Work out the finished part from the listing and answer in its coordinate system (mm). Face numbers are marked on the shaded views. A direction names the side the tool comes from. Coordinates: 2 decimals unless noted, no trailing zeros. Write each loop counter-clockwise with the first axis right and the second up, starting at its lowest first coordinate (ties: lowest second). Pieces come first, ordered by that corner, then holes. Notation, with made-up numbers: (83, -34) - (119, -34) arc R27 cw to (119, 1) - close; hole circle Ø8 at (-39, -2.5). An arc over 180 degrees is marked (long way). Use CSV: the item, a comma, the result in double quotes. Start each with the question number.
from build123d import *

# Parameters (mm, degrees)
SKETCH2_R           = 16
BOSS_EXTRUDE1_DEPTH = 5
SKETCH3_R           = 7.5
BOSS_EXTRUDE2_DEPTH = 19
SKETCH4_R           = 4
CUT_EXTRUDE1_DEPTH  = 50
SKETCH5_R           = 2
CUT_EXTRUDE2_DEPTH  = 50


with BuildPart() as part:
    # Sketch2 → Boss-Extrude1 (new body)
    with BuildSketch(Plane(origin=(0, 0, 0), x_dir=(1, 0, 0), z_dir=(0, 1, 0))):
        Circle(SKETCH2_R)
    extrude(amount=BOSS_EXTRUDE1_DEPTH)

    # Sketch3 → Boss-Extrude2 (add)
    with BuildSketch(Plane(origin=(0, 5, 0), x_dir=(1, 0, 0), z_dir=(0, 1, 0))):
        Circle(SKETCH3_R)
    extrude(amount=BOSS_EXTRUDE2_DEPTH)

    # Sketch4 → Cut-Extrude1 (cut)
    with BuildSketch(Plane(origin=(0, 24, 0), x_dir=(1, 0, 0), z_dir=(0, 1, 0))):
        Circle(SKETCH4_R)
    extrude(amount=-CUT_EXTRUDE1_DEPTH, mode=Mode.SUBTRACT)

    # Sketch5 → Cut-Extrude2 (cut)
    with BuildSketch(Plane(origin=(0, 5, 0), x_dir=(1, 0, 0), z_dir=(0, 1, 0))):
        with Locations((0, 12)):
            Circle(SKETCH5_R)
        with Locations((0, -12)):
            Circle(SKETCH5_R)
        with Locations((-12, 0)):
            Circle(SKETCH5_R)
        with Locations((12, 0)):
            Circle(SKETCH5_R)
    extrude(amount=-CUT_EXTRUDE2_DEPTH, mode=Mode.SUBTRACT)


solid = part.part
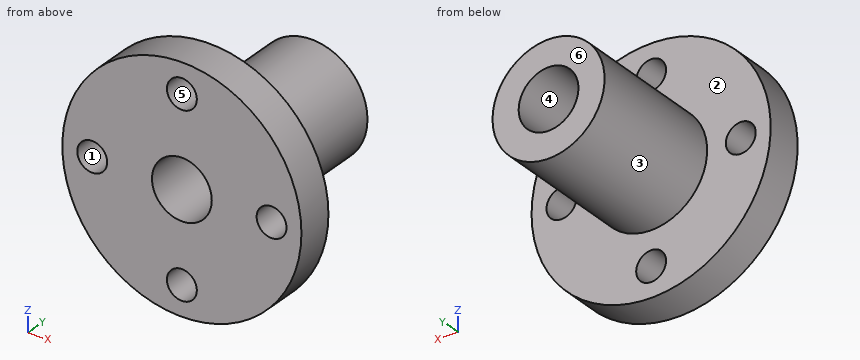
Item 1: Each of these flat-tipped pins is pushed along its axis until it touches: pin 1 (6 mm diameter, centred on x = 7.5, y = 19, fed in from -Z); pin 2 (8 mm diameter, centred on x = -7, y = 14, fed in from -Z); pin 3 (4.5 mm diameter, centred on x = 0, z = -12, fed in from +Y). Where does it stop, or does it pass through?
Item 2: Straight lines are drawn through the part: probe 1 along X at (y, z) = (2.85, 0); probe 2 along X at (y, z) = (6, 0). For each, find the intervals that lie inside material, in ascending order. Write a range as [from, to].
Item 3: A cutting plane is placed at C-C (x = -12). Determine the outline of the cut face in (y, z).
Item 4: Which of the six approach directions +Z, -Z, +X, -X, +Y, -Y give full straight-line access (tool end or side, diameter ignored) to the marked faces 1 and 2?
Item 5: A cutting plane is placed at A-A (x = 0). Determine the outline of the cut face in (y, z).
Item 6: A cutting plane is placed at D-D (y = 7.75). Determine the outline of the cut face in (x, z), then the cut area to 3 significant figures.
Item 7: A cutting plane is placed at B-B (z = 0.5). Determine the outline of the cut face in (x, y), then the cut area to 3 significant figures.
Item 8: Determine the mould class of the marked faces 3, 4, 5 and 6 for opening direction X: +X half, -X half, draft (parallel to the pull), parting line (faces both ways), or undercut.
Calculated:
1,pin 1,"stops at z = -6"
1,pin 2,"stops at z = -6.87"
1,pin 3,"stops at y = 5"
2,probe 1,"x = [-16, -14], [-10, -4], [4, 10], [14, 16]"
2,probe 2,"x = [-7.5, -4], [4, 7.5]"
3,outline,"(0, -10.58) - (5, -10.58) - (5, -2) - (0, -2) - close; (0, 2) - (5, 2) - (5, 10.58) - (0, 10.58) - close"
4,face 1,"+Y, -Y"
4,face 2,"+Y"
5,outline,"(0, -16) - (5, -16) - (5, -14) - (0, -14) - close; (0, -10) - (5, -10) - (5, -7.5) - (24, -7.5) - (24, -4) - (0, -4) - close; (0, 4) - (24, 4) - (24, 7.5) - (5, 7.5) - (5, 10) - (0, 10) - close; (0, 14) - (5, 14) - (5, 16) - (0, 16) - close"
6,outline,"circle Ø15 at (0, 0); hole circle Ø8 at (0, 0)"
6,area,"126 mm²"
7,outline,"(-15.99, 0) - (-13.94, 0) - (-13.94, 5) - (-15.99, 5) - close; (-10.06, 0) - (-3.97, 0) - (-3.97, 24) - (-7.48, 24) - (-7.48, 5) - (-10.06, 5) - close; (3.97, 0) - (10.06, 0) - (10.06, 5) - (7.48, 5) - (7.48, 24) - (3.97, 24) - close; (13.94, 0) - (15.99, 0) - (15.99, 5) - (13.94, 5) - close"
7,area,"215 mm²"
8,face 3,"parting line"
8,face 4,"undercut"
8,face 5,"undercut"
8,face 6,"draft"
